Here's how the part is built. I have some questions about the finished solid (model axes, mm). Coordinates: 2 decimals unless noted, no trailing zeros. Write each loop counter-clockwise with the first axis right and the second up, starting at its lowest first coordinate (ties: lowest second). Pieces come first, ordered by that corner, then holes. Notation, with made-up numbers: (12.25, 4.25) -> (24.25, 4.25) arc R11 ccw to (24.25, 21.25) -> close; hole circle Ø9 at (66.25, 4.5). An arc over 180 degrees is marked (long way). Put each result on its own line as item: value.
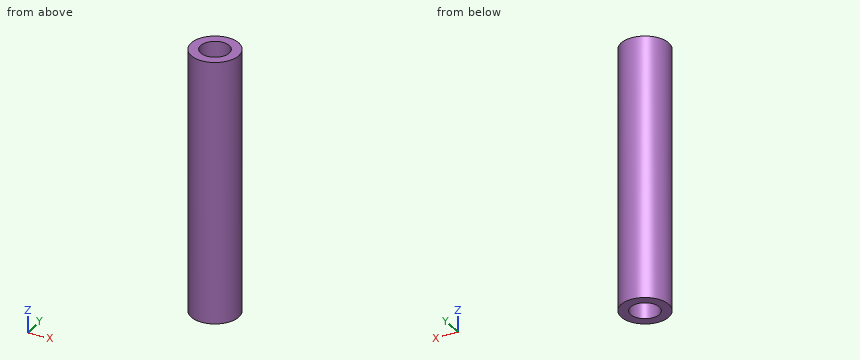
```python
from build123d import *

# Parameters (mm, degrees)
BOSS_EXTRUDE1_DEPTH      = 25
BOSS_EXTRUDE1_DEPTH_BACK = 2.5
SKETCH1_R                = 2.5
SKETCH3_R                = 1.5
CUT_EXTRUDE1_DEPTH       = 6
CUT_EXTRUDE2_START       = -6
SKETCH2_R                = 1.5
CUT_EXTRUDE2_DEPTH       = 6


with BuildPart() as part:
    # Sketch1 → Boss-Extrude1 (new, two sides: drawn at the far end of the back side and taken through both)
    with BuildSketch(Plane.XY.offset(-BOSS_EXTRUDE1_DEPTH_BACK)):
        Circle(SKETCH1_R)
    extrude(amount=BOSS_EXTRUDE1_DEPTH + BOSS_EXTRUDE1_DEPTH_BACK)

    # Sketch3 → Cut-Extrude1 (cut)
    with BuildSketch(Plane(origin=(0, 0, -2.5), x_dir=(-1, 0, 0), z_dir=(0, 0, -1))):
        Circle(SKETCH3_R)
    extrude(amount=-CUT_EXTRUDE1_DEPTH, mode=Mode.SUBTRACT)

    # Sketch2 → Cut-Extrude2 (cut)
    with BuildSketch(Plane.XY.offset(25).offset(CUT_EXTRUDE2_START)):
        with Locations(Location((0, 0, 0), (0, 0, 180))):
            Circle(SKETCH2_R)
    extrude(amount=CUT_EXTRUDE2_DEPTH, mode=Mode.SUBTRACT)


solid = part.part
```
Item 1: Imagine slicing it at A-A on x = 0. Write out the boundary of the cut face in (y, z), then the cut area to 4 significant figures.
Output:
outline: (-2.5, -2.5) -> (-1.5, -2.5) -> (-1.5, 3.5) -> (1.5, 3.5) -> (1.5, -2.5) -> (2.5, -2.5) -> (2.5, 25) -> (1.5, 25) -> (1.5, 19) -> (-1.5, 19) -> (-1.5, 25) -> (-2.5, 25) -> close
area: 101.5 mm²
Item 2: Please list where these lines run through material, in increasing order: line 1 along Y through (x, z) = (0, 0.3); line 2 along X through (y, z) = (-0.1, 17.75); line 3 along Y through (x, z) = (-0.5, 3.25). Write a range as from..to.
Output:
line 1: y = -2.5..-1.5, 1.5..2.5
line 2: x = -2.5..2.5
line 3: y = -2.45..-1.41, 1.41..2.45
Item 3: Imagine slicing it at C-C on z = 22.75. Write out the boundary of the cut face in (x, y).
Output:
outline: circle Ø5 at (0, 0); hole circle Ø3 at (0, 0)
Item 4: For P1, Ø2.5, axis at x = 0, y = 0, coming from the -Z side; P2, Ø1.5, axis at x = 0, y = -0.5, coming from the +Z side; P3, Ø1.5, axis at y = 1, z = 9.5, coming from the +X side, each with a flat end and sliding along its axis, tell me the tip position at first contact or that it passes through.
Output:
P1: stops at z = 3.5
P2: stops at z = 19
P3: stops at x = 2.49
Item 5: Imagine slicing it at D-D on z = 16. Write out the boundary of the cut face in (x, y).
Output:
outline: circle Ø5 at (0, 0)
